Could you check a few things on this model? Use its own coordinates, in mm. A direction names the side the tool comes from. Coordinates: 2 decimals unless noted, no trailing zeros. Loops run counter-clockwise (first coordinate to the right, second up) from the corner with the lowest first, then second, coordinate; pieces in that order, holes last.
1) Imagine slicing it at C-C on x = -535. Please give me the cut outline in (y, z), plus the area to 3 significant figures.
2) Imagine slicing it at A-A on z = -159.5. Please give me the cut outline in (x, y).
3) Thinking about a two-plate mould opening in X: for faces 4 (the face through (600, -544, -1)), 5 (the face through (250, -49, -4)), 6 (the face through (-250, -49, -4)), 7 (the face through (-14, 250, -7)), which applies, released by +X, released by -X, zero draft, split by the parting line, or undercut?
4) If I drill on line 1 along X through (y, z) = (-9, -90); line 2 along Y through (x, z) = (538.5, 353); line 3 along Y through (x, z) = (317.5, -54.5), over which ranges is the centre line in solid material (lowest first)?
5) Imagine slicing it at B-B on x = 522.5. Please give me the cut outline in (y, z), plus the area to 3 significant figures.
6) For faces 1 (the face through (-504, -49, -251.581)), 2 (the face through (750, -49, -4)), 3 (the face through (-750, -49, -4)), which set-ups out of +Z, -Z, +X, -X, +Y, -Y let a thin tool reach every point of the face, with its end or its side?
7) Will these pins go through, and if not, where does the flat tip stop? P1, Ø2, axis at y = -99, z = 147.5, coming from the +X side; P2, Ø5, axis at x = -525, z = -26, coming from the -Y side; P3, Ø2, axis at x = -324, y = -63.5, coming from the -Z side.
8) Imagine slicing it at D-D on y = -167.5. Please give me the cut outline in (x, z).
```python
from build123d import *

# Parameters (mm, degrees)
SKETCH2_W           = 2000
SKETCH2_H           = 1000
BOSS_EXTRUDE1_DEPTH = 250
SKETCH3_W           = 500
SKETCH3_H           = 503.161668984
BOSS_EXTRUDE2_DEPTH = 100
SKETCH4_W           = 200
SKETCH4_H           = 201.264667594
BOSS_EXTRUDE3_DEPTH = 900


with BuildPart() as part:
    # Sketch2 → Boss-Extrude1 (new body)
    with BuildSketch(Plane(origin=(0, 0, 0), x_dir=(1, 0, 0), z_dir=(0, 1, 0))):
        Rectangle(SKETCH2_W, SKETCH2_H)
    extrude(amount=BOSS_EXTRUDE1_DEPTH)

    # Sketch3 → Boss-Extrude2 (add)
    with BuildSketch(Plane.XZ):
        with Locations((-500, 0)):
            Rectangle(SKETCH3_W, SKETCH3_H)
        with Locations((500, 0)):
            Rectangle(SKETCH3_W, SKETCH3_H)
    extrude(amount=BOSS_EXTRUDE2_DEPTH)

    # Sketch4 → Boss-Extrude3 (add)
    with BuildSketch(Plane.XZ.offset(100)):
        with Locations((500, 0)):
            Rectangle(SKETCH4_W, SKETCH4_H)
    extrude(amount=BOSS_EXTRUDE3_DEPTH)


solid = part.part
```
Filled in:
1. outline: (-100, -251.58) - (0, -251.58) - (0, -500) - (250, -500) - (250, 500) - (0, 500) - (0, 251.58) - (-100, 251.58) - close
1. area: 300,000 mm2
2. outline: (-1000, 0) - (-750, 0) - (-750, -100) - (-250, -100) - (-250, 0) - (250, 0) - (250, -100) - (750, -100) - (750, 0) - (1000, 0) - (1000, 250) - (-1000, 250) - close
3. face 4: released by +X
3. face 5: undercut
3. face 6: undercut
3. face 7: zero draft
4. line 1: x = -750 to -250, 250 to 750
4. line 2: y = 0 to 250
4. line 3: y = -100 to 250
5. outline: (-1000, -100.63) - (-100, -100.63) - (-100, -251.58) - (0, -251.58) - (0, -500) - (250, -500) - (250, 500) - (0, 500) - (0, 251.58) - (-100, 251.58) - (-100, 100.63) - (-1000, 100.63) - close
5. area: 481,000 mm2
6. face 1: -Z, +X, -X, -Y
6. face 2: +Z, -Z, +X, -Y
6. face 3: +Z, -Z, -X, -Y
7. P1: stops at x = 750
7. P2: stops at y = -100
7. P3: stops at z = -251.58
8. outline: (400, -100.63) - (600, -100.63) - (600, 100.63) - (400, 100.63) - close
